Build history of the part. All positions in model axes, mm. A direction names the side the tool comes from. Coordinates: 2 decimals unless noted, no trailing zeros. Loops run counter-clockwise (first coordinate to the right, second up) from the corner with the lowest first, then second, coordinate; pieces in that order, holes last.
Item 1: Cut at A-A (z = -62). List the corners of the cut face in (x, y).
Item 2: Drill centre lines: line 1 along Z through (x, y) = (28, 0); line 2 along Y through (x, z) = (68, -50.5); line 3 along Y through (x, z) = (116, -33). Where is each one in solid material? Low to high.
Item 3: Mould opens along X. For faces 1 (the face through (-2, 7, 0)), 2 (the face through (25.16, 4.73, -40.43)), 3 (the face through (95, 0, -82)), 4 (the face through (155, 0, 10)) say: released by +X, released by -X, zero draft, split by the parting line, or undercut.
Item 4: Cut at C-C (x = 72.5). List the corners of the cut face in (y, z).
Item 5: Cut at B-B (x = 145). List the corners of the cut face in (y, z), and give its area (3 significant figures).
Item 6: 3-axis set-ups, long thin cutter, end or side, ignore diameter. For faces 5 (the face through (102, 0, -40)), 6 (the face through (-2, -8.25, 10)): which of +Z, -Z, +X, -X, +Y, -Y reach the whole face in a straight line?
Item 7: Flat gauge pins, fed straight in: pin 1 (4 mm diameter, centred on y = -4, z = -62.5, fed in from -X); pin 2 (5 mm diameter, centred on y = 1.5, z = -38, fed in from -X); pin 3 (3 mm diameter, centred on y = -1.5, z = -59.5, fed in from +X). Where does each tip first touch, or does it go through?
from build123d import *

# Parameters (mm, degrees)
SKETCH2_W           = 310
SKETCH2_H           = 16.5
BOSS_EXTRUDE1_DEPTH = 20
SKETCH3_R           = 7
BOSS_EXTRUDE2_DEPTH = 82
LPATTERN1_COUNT     = 8
LPATTERN1_PITCH     = 25


with BuildPart() as part:
    # Sketch2 → Boss-Extrude1 (new body)
    with BuildSketch(Plane.XY):
        Rectangle(SKETCH2_W, SKETCH2_H)
    extrude(amount=BOSS_EXTRUDE1_DEPTH)

    # Sketch3 → Boss-Extrude2 (add)
    with BuildSketch(Plane(origin=(0, 0, 0), x_dir=(-1, 0, 0), z_dir=(0, 0, -1))):
        with Locations((-145, 0)):
            Circle(SKETCH3_R)
    boss_extrude2 = extrude(amount=BOSS_EXTRUDE2_DEPTH)

    # LPattern1: Boss-Extrude2 ×8
    with Locations(*[(-i * LPATTERN1_PITCH, 0, 0) for i in range(1, LPATTERN1_COUNT)]):
        add(boss_extrude2)


solid = part.part
Filled sheet:
1. outline: circle Ø14 at (-30, 0); circle Ø14 at (-5, 0); circle Ø14 at (20, 0); circle Ø14 at (45, 0); circle Ø14 at (70, 0); circle Ø14 at (95, 0); circle Ø14 at (120, 0); circle Ø14 at (145, 0)
2. line 1: z = 0 to 20
2. line 2: y = -6.71 to 6.71
2. line 3: y = -5.74 to 5.74
3. face 1: undercut
3. face 2: undercut
3. face 3: zero draft
3. face 4: released by +X
4. outline: (-8.25, 0) - (-6.54, 0) - (-6.54, -82) - (6.54, -82) - (6.54, 0) - (8.25, 0) - (8.25, 20) - (-8.25, 20) - close
5. outline: (-8.25, 0) - (-7, 0) - (-7, -82) - (7, -82) - (7, 0) - (8.25, 0) - (8.25, 20) - (-8.25, 20) - close
5. area: 1,480 mm2
6. face 5: -Z
6. face 6: +Z, -Z, +X, -X, -Y
7. pin 1: stops at x = -36.71
7. pin 2: stops at x = -37
7. pin 3: stops at x = 152
